Input: part model. Units: mm. Frame: model coordinates. Face numbers are marked on the shaded views. A direction names the side the tool comes from. Give positions to 0.01 mm unless a question says otherwise; leave off trailing zeros. Write each loop counter-clockwise with the first axis right and the second up, starting at its lowest first coordinate (ties: lowest second). Pieces come first, ordered by that corner, then holes. Notation, with made-up numbers: (1, 71.5) - (55, 71.5) arc R24 ccw to (55, 107.5) - close; hole circle Ø4 at (17, 49). An arc over 180 degrees is marked (long way). Answer as CSV lines item,"result".
```python
from build123d import *

# Parameters (mm, degrees)
SKETCH_R     = 20.5
PAD_DEPTH    = 1
SKETCH002_R  = 1.95
HOLE_DEPTH   = 1.001
SKETCH003_R  = 4
PAD001_DEPTH = 5.5
POCKET_DEPTH = 5.501


with BuildPart() as part:
    # Sketch → Pad (new body)
    with BuildSketch(Plane.XY):
        with Locations((20.5, 20.5)):
            Circle(SKETCH_R)
    extrude(amount=PAD_DEPTH)

    # Sketch002 → Hole (cut, through all)
    with BuildSketch(Plane.XY):
        with Locations((9.75, 4.5)):
            Circle(SKETCH002_R)
        with Locations((31.25, 4.5)):
            Circle(SKETCH002_R)
        with Locations((20.5, 39.5)):
            Circle(SKETCH002_R)
    extrude(amount=HOLE_DEPTH, mode=Mode.SUBTRACT)

    # Sketch003 → Pad001 (join, symmetric)
    with BuildSketch(Plane.XY):
        with Locations((20.5, 20.5)):
            Circle(SKETCH003_R)
    extrude(amount=PAD001_DEPTH, both=True)

    # Sketch004 → Pocket (cut, through all)
    with BuildSketch(Plane.XY):
        with BuildLine():
            Line((18.65, 22.796447), (18.65, 18.203553))
            ThreePointArc((18.65, 18.203553), (18.753553, 17.953553), (19.003553, 17.85))
            Line((19.003553, 17.85), (21.996447, 17.85))
            ThreePointArc((21.996447, 17.85), (22.246447, 17.953553), (22.35, 18.203553))
            Line((22.35, 18.203553), (22.35, 22.796447))
            ThreePointArc((22.35, 22.796447), (22.246447, 23.046447), (21.996447, 23.15))
            Line((21.996447, 23.15), (19.003553, 23.15))
            ThreePointArc((19.003553, 23.15), (18.753553, 23.046447), (18.65, 22.796447))
        make_face()
    extrude(amount=POCKET_DEPTH, mode=Mode.SUBTRACT)


solid = part.part
```
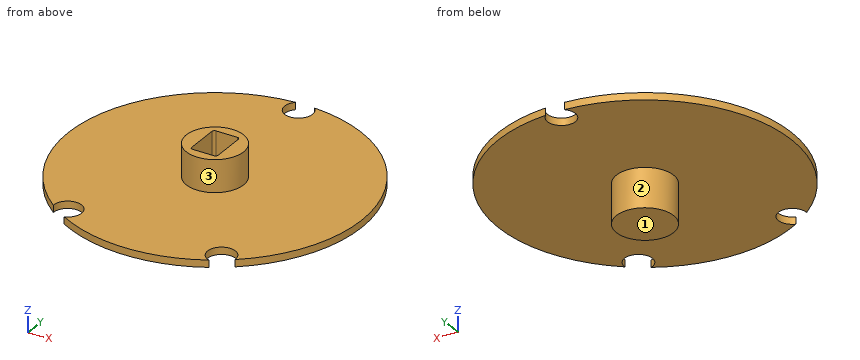
Item 1: Cut plane B-B on z = 1.75. Return the cut outline in (x, y), plus the area to 3 significant figures.
The answers:
outline,"circle Ø8 at (20.5, 20.5); hole (18.65, 18.2) arc R0.35 ccw to (19, 17.85) - (22, 17.85) arc R0.35 ccw to (22.35, 18.2) - (22.35, 22.8) arc R0.35 ccw to (22, 23.15) - (19, 23.15) arc R0.35 ccw to (18.65, 22.8) - close"
area,"30.8 mm²"
Item 2: Cut plane A-A on y = 5. Return the cut outline in (x, z).
The answers:
outline,"(7.08, 0) - (7.87, 0) - (7.87, 1) - (7.08, 1) - close; (11.63, 0) - (29.37, 0) - (29.37, 1) - (11.63, 1) - close; (33.13, 0) - (33.92, 0) - (33.92, 1) - (33.13, 1) - close"
Item 3: Cut plane D-D on y = 20.5. Return the cut outline in (x, z), plus the area to 3 significant figures.
The answers:
outline,"(0, 0) - (16.5, 0) - (16.5, -5.5) - (24.5, -5.5) - (24.5, 0) - (41, 0) - (41, 1) - (24.5, 1) - (24.5, 5.5) - (22.35, 5.5) - (22.35, 0) - (18.65, 0) - (18.65, 5.5) - (16.5, 5.5) - (16.5, 1) - (0, 1) - close"
area,"101 mm²"
Item 4: Contact query for flat-ended pins moving along their axis: pin 1 (6 mm diameter, centred on x = 20.5, y = 39.5, fed in from +Z); pin 2 (3.5 mm diameter, centred on y = 20.5, z = 4, fed in from -X); pin 3 (8 mm diameter, centred on x = 12.5, y = 22, fed in from -Z). Output: stop coordinate, or through.
The answers:
pin 1,"z = 1"
pin 2,"x = 16.5"
pin 3,"z = 0"
Item 5: Cut plane C-C on x = 20.5. Return the cut outline in (y, z).
The answers:
outline,"(0, 0) - (16.5, 0) - (16.5, -5.5) - (24.5, -5.5) - (24.5, 0) - (37.55, 0) - (37.55, 1) - (24.5, 1) - (24.5, 5.5) - (23.15, 5.5) - (23.15, 0) - (17.85, 0) - (17.85, 5.5) - (16.5, 5.5) - (16.5, 1) - (0, 1) - close"
Item 6: Ray query, line 1 (Z direction, x = 16.5, y = 2); line 2 (X direction, y = 38.5, z = 0.5); line 3 (X direction, y = 14, z = 0.5). Return the intervals inside material, ascending. Write a range as from..to.
The answers:
line 1,"0..1"
line 2,"10.69..18.83, 22.17..30.31"
line 3,"1.06..39.94"
Item 7: Reachability of the marked faces 1, 2 and 3 from +Z, -Z, +X, -X, +Y, -Y: full face, straight path, thin tool, end or side. Return the list, or none.
The answers:
face 1,"-Z, +X, -X, +Y, -Y"
face 2,"-Z"
face 3,"+Z"
